Check sheet for the modelled part. Datum: model origin and axes. Units: mm. A direction names the side the tool comes from. Round coordinates to 2 decimals unless told otherwise and drop trailing zeros. Order: outer loops, then holes, each group sorted by start corner. A loop starts at its lowest first (then second) coordinate and runs counter-clockwise, first axis right, second up.
from build123d import *

# Parameters (mm, degrees)
SKETCH047_R      = 5
EXTRUDE030_DEPTH = 5
SKETCH045_R      = 12
EXTRUDE028_DEPTH = 7
SKETCH042_R      = 4
EXTRUDE025_DEPTH = 30
SKETCH040_R      = 7
SKETCH043_W      = 60
SKETCH043_H      = 15
EXTRUDE026_DEPTH = 150


with BuildPart() as extrude030:
    # Sketch047 → Extrude030 (new body)
    with BuildSketch(Plane.XY):
        with Locations((19.376185, 19.084115)):
            Circle(SKETCH047_R)
        with Locations((114.867691, -14.293477)):
            Circle(SKETCH047_R)
    extrude(amount=EXTRUDE030_DEPTH)


with BuildPart() as sprue_and_vent001:
    # Sketch045 → Extrude028 (new body)
    with BuildSketch(Plane.XY.offset(15)):
        with Locations((29.491073, -5.076964)):
            Circle(SKETCH045_R)
        with Locations((104.246048, 7.486251)):
            Circle(SKETCH045_R)
    extrude(amount=-EXTRUDE028_DEPTH)


with BuildPart() as sweep012:
    # Sweep012: sweep along a path in Sketch
    with BuildLine(Plane.XY) as sweep012_path:
        ThreePointArc((0, 0), (65.583227, -3.22849), (127, 20))
    # Sketch042 → Sweep012 (sweep)
    with BuildSketch(Plane(origin=(0, 0, 0), x_dir=(0, -1, 0), z_dir=(-1, 0, 0))):
        Circle(SKETCH042_R)
    sweep(path=sweep012_path.line)


with BuildPart() as sweep012_1:
    # Sweep012 placement: moved
    add(sweep012.part.moved(Location((0, -3, 0))))


with BuildPart() as extrude025:
    # Sketch041 → Extrude025 (new body)
    with BuildSketch(Plane.XY.offset(-15)):
        Polygon((-8.268976, 21.973037), (10.121624, 21.973037), (-0.555824, -25), (-25.401805, -25), align=None)
        Polygon((105.81268, 45.885295), (155.276998, 45.885295), (207.473539, -4.114705), (135.506671, -4.114705), align=None)
    extrude(amount=EXTRUDE025_DEPTH)


with BuildPart() as fusion012:
    # Sweep009: sweep along a path in Sketch
    with BuildLine(Plane.XY) as sweep009_path:
        ThreePointArc((0, 0), (65.583227, -3.22849), (127, 20))
    # Sketch040 → Sweep009 (sweep)
    with BuildSketch(Plane(origin=(0, 0, 0), x_dir=(0, -1, 0), z_dir=(-1, 0, 0))):
        Circle(SKETCH040_R)
    sweep(path=sweep009_path.line)

    # Cut011: cut Extrude025
    add(extrude025.part, mode=Mode.SUBTRACT)

    # Fusion011: union Sweep012
    add(sweep012_1.part)

    # Fusion012: union Sprue and Vent001
    add(sprue_and_vent001.part)


with BuildPart() as motor_mold_top:
    # Sketch043 → Extrude026 (new body)
    with BuildSketch(Plane(origin=(-10, 0, 0), x_dir=(0, -1, 0), z_dir=(-1, 0, 0))):
        with Locations((-2, 7.5)):
            Rectangle(SKETCH043_W, SKETCH043_H)
    extrude(amount=-EXTRUDE026_DEPTH)

    # Cut012: cut Fusion012
    add(fusion012.part, mode=Mode.SUBTRACT)

    # Cut014: cut Extrude030
    add(extrude030.part, mode=Mode.SUBTRACT)


solid = motor_mold_top.part
1) Sectioned sample at B-B on z = 2.25. Count the separate pieces of the cut face and the enclosed holes in it, and give its area (3 significant figures).
2) Sectioned sample at A-A on z = 9.5. Record the cut outline in (x, y).
3) Gauge pin test, flat ends, axial feed: pin 1 (3 mm diameter, centred on x = 21, y = 17, fed in from -Z); pin 2 (19 mm diameter, centred on x = 103.5, y = 7, fed in from +Z). Record the tip position at first contact, or that the pin passes through.
4) Scan lines: line 1 (X direction, y = 1, z = 10); line 2 (Y direction, x = 19, z = 10); line 3 (X direction, y = 8, z = 12.5). Record each from-to range of solid material in increasing order.
5) Draft check along Y on faces 1 (the face through (122.03, 18.58, 3.46)), 2 (the face through (64, -28, 7)), 3 (the face through (64, 2, 15)). Enter one of: pulls with the +Y half, pulls with the -Y half, needs draft (parallel to the pull), parting line crosses it, or undercut.
6) Set-up check for faces 4 (the face through (115, -14, 5)), 5 (the face through (92.258, 8.014, 11.549)), 6 (the face through (64, 32, 7)): record each of +Z, -Z, +X, -X, +Y, -Y from which the full face is reachable in a straight line by a thin tool's end or side.
Values found:
1. separate pieces: 1
1. enclosed holes: 3
1. area: 7,220 mm2
2. outline: (-10, -28) - (140, -28) - (140, 32) - (-10, 32) - close; hole circle Ø24 at (29.49, -5.08); hole circle Ø24 at (104.25, 7.49)
3. pin 1: stops at z = 5
3. pin 2: stops at z = 8
4. line 1: x = -10 to 19.14, 39.84 to 94.15, 114.34 to 140
4. line 2: y = -28 to -10.9, 0.75 to 32
4. line 3: x = -10 to 92.26, 116.24 to 140
5. face 1: undercut
5. face 2: pulls with the -Y half
5. face 3: needs draft
6. face 4: -Z
6. face 5: +Z
6. face 6: +Z, -Z, +X, -X, +Y
